from build123d import *

# Parameters (mm, degrees)
F1_DEPTH = 3
F2_R     = 5
F0_W     = 3
F0_H     = 6.5
F3_DEPTH = 7
F4_R     = 0.95
F5_DEPTH = 25
F6_R     = 1.99999


# Not quite as in the source:
# - a fillet or chamfer is up to 0.001 mm smaller than in the source, because OpenCascade refuses the exact size
# - a feature names something its author has since deleted; it is built from what else it names


with BuildPart() as f1:
    # F0 (on Top) → F1 (new body)
    with BuildSketch(Plane.XY):
        with BuildLine():
            Line((-23.06675, 0), (-28.2842712475, 0))
            Line((-28.2842712475, 0), (0, -28.2842712475))
            Line((0, -28.2842712475), (0, -23.0667636524))
            ThreePointArc((0, -23.0667636524), (-1.5, -21.5667636524), (0, -20.0667636524))
            Line((0, -20.0667636524), (0, -14.2842712475))
            Line((0, -14.2842712475), (-4.5, -14.2842712475))
            Line((-4.5, -14.2842712475), (-7.5, -14.2842712475))
            Line((-7.5, -14.2842712475), (-7.5, -7.7842712475))
            Line((-7.5, -7.7842712475), (-7.5, 0))
            Line((-7.5, 0), (-20.06675, 0))
            ThreePointArc((-20.06675, 0), (-21.56675, -1.5), (-23.06675, 0))
        make_face()
        with BuildLine():
            Line((0, -23.0667636524), (0, -28.2842712475))
            Line((0, -28.2842712475), (28.2842712475, 0))
            Line((28.2842712475, 0), (23.06675, 0))
            ThreePointArc((23.06675, 0), (21.56675, -1.5), (20.06675, 0))
            Line((20.06675, 0), (7.5, 0))
            Line((7.5, 0), (7.5, -7.7842712475))
            Line((7.5, -7.7842712475), (7.5, -14.2842712475))
            Line((7.5, -14.2842712475), (4.5, -14.2842712475))
            Line((4.5, -14.2842712475), (0, -14.2842712475))
            Line((0, -14.2842712475), (0, -20.0667636524))
            ThreePointArc((0, -20.0667636524), (1.0606601718, -20.5061034806), (1.5, -21.5667636524))
            ThreePointArc((1.5, -21.5667636524), (1.0606601718, -22.6274238242), (0, -23.0667636524))
        make_face()
        with BuildLine():
            Line((-4.2426406871, 24.0416305603), (-28.2842712475, 0))
            Line((-28.2842712475, 0), (-23.06675, 0))
            ThreePointArc((-23.06675, 0), (-21.56675, 1.5), (-20.06675, 0))
            Line((-20.06675, 0), (-7.5, 0))
            Line((-7.5, 0), (-7.5, 4.6038874425))
            Line((-7.5, 4.6038874425), (0, 4.6038874425))
            Line((0, 4.6038874425), (0, 20.0667636524))
            ThreePointArc((0, 20.0667636524), (-1.3266484173, 20.8667608118), (-1.2382102141, 22.4134250167))
            ThreePointArc((-1.2382102141, 22.4134250167), (-2.8587925726, 23.0091120056), (-4.2426406871, 24.0416305603))
        make_face()
        with BuildLine():
            ThreePointArc((0, 34.2842712475), (-5.5432771951, 30.5803718417), (-4.2426406871, 24.0416305603))
            Line((-4.2426406871, 24.0416305603), (-2.2273863607, 26.0568848867))
            ThreePointArc((-2.2273863607, 26.0568848867), (-2.9102205274, 29.4897240594), (0, 31.4342712475))
            Line((0, 31.4342712475), (0, 34.2842712475))
        make_face()
        with BuildLine():
            Line((-2.2273863607, 26.0568848867), (-4.2426406871, 24.0416305603))
            ThreePointArc((-4.2426406871, 24.0416305603), (-2.8587925726, 23.0091120056), (-1.2382102141, 22.4134250167))
            ThreePointArc((-1.2382102141, 22.4134250167), (-0.7000028406, 22.8934120697), (0, 23.0667636524))
            Line((0, 23.0667636524), (0, 25.1342712475))
            ThreePointArc((0, 25.1342712475), (-1.205452812, 25.3740507201), (-2.2273863607, 26.0568848867))
        make_face()
        with BuildLine():
            ThreePointArc((6, 28.2842712475), (4.2426406871, 32.5269119346), (0, 34.2842712475))
            Line((0, 34.2842712475), (0, 31.4342712475))
            ThreePointArc((0, 31.4342712475), (2.2273863607, 30.5116576082), (3.15, 28.2842712475))
            ThreePointArc((3.15, 28.2842712475), (2.9102205274, 27.0788184355), (2.2273863607, 26.0568848867))
            Line((2.2273863607, 26.0568848867), (4.2426406871, 24.0416305603))
            ThreePointArc((4.2426406871, 24.0416305603), (5.5432771951, 25.9881706533), (6, 28.2842712475))
        make_face()
        with BuildLine():
            ThreePointArc((1.2382102141, 22.4134250167), (2.8587925726, 23.0091120056), (4.2426406871, 24.0416305603))
            Line((4.2426406871, 24.0416305603), (2.2273863607, 26.0568848867))
            ThreePointArc((2.2273863607, 26.0568848867), (1.2054528119, 25.3740507201), (0, 25.1342712475))
            Line((0, 25.1342712475), (0, 23.0667636524))
            ThreePointArc((0, 23.0667636524), (0.7000028406, 22.8934120697), (1.2382102141, 22.4134250167))
        make_face()
        with BuildLine():
            Line((23.06675, 0), (28.2842712475, 0))
            Line((28.2842712475, 0), (4.2426406871, 24.0416305603))
            ThreePointArc((4.2426406871, 24.0416305603), (2.8587925726, 23.0091120056), (1.2382102141, 22.4134250167))
            ThreePointArc((1.2382102141, 22.4134250167), (1.4330588476, 22.0098689891), (1.5, 21.5667636524))
            ThreePointArc((1.5, 21.5667636524), (1.0606601718, 20.5061034806), (0, 20.0667636524))
            Line((0, 20.0667636524), (0, 4.6038874425))
            Line((0, 4.6038874425), (7.5, 4.6038874425))
            Line((7.5, 4.6038874425), (7.5, 0))
            Line((7.5, 0), (20.06675, 0))
            ThreePointArc((20.06675, 0), (21.56675, 1.5), (23.06675, 0))
        make_face()
    extrude(amount=F1_DEPTH)

    # F2
    f2_edges = [f1.edges().sort_by_distance(p)[0] for p in [
        (-28.284271, 0, 1.5),
        (28.284271, 0, 1.5),
        (0, -28.284271, 1.5),
        (4.242641, 24.041631, 1.5),
        (-4.242641, 24.041631, 1.5),
    ]]
    fillet(f2_edges, radius=F2_R)

    # F0 (on Top) → F3 (join)
    with BuildSketch(Plane.XY):
        with Locations((-6, -11.0342712475)):
            Rectangle(F0_W, F0_H)
        with Locations((6, -11.0342712475)):
            Rectangle(F0_W, F0_H)
    extrude(amount=F3_DEPTH)

    # F4 (on face) → F5 (cut)
    with BuildSketch(Plane(origin=(-7.5, 0, 0), x_dir=(0, -1, 0), z_dir=(-1, 0, 0))):
        with Locations((11.0342712475, 5.05)):
            Circle(F4_R)
    extrude(amount=-F5_DEPTH, mode=Mode.SUBTRACT)

    # F6 (radius 2 in the source; OpenCascade refuses exactly that, so slightly less here)
    f6_edges = [f1.edges().sort_by_distance(p)[0] for p in [
        (-6, -14.284271, 7),
        (-6, -14.284271, 3),
        (-6, -7.784271, 7),
        (-6, -7.784271, 0),
        (6, -7.784271, 0),
        (6, -14.284271, 3),
        (6, -14.284271, 7),
        (6, -7.784271, 7),
    ]]
    fillet(f6_edges, radius=F6_R)


solid = f1.part
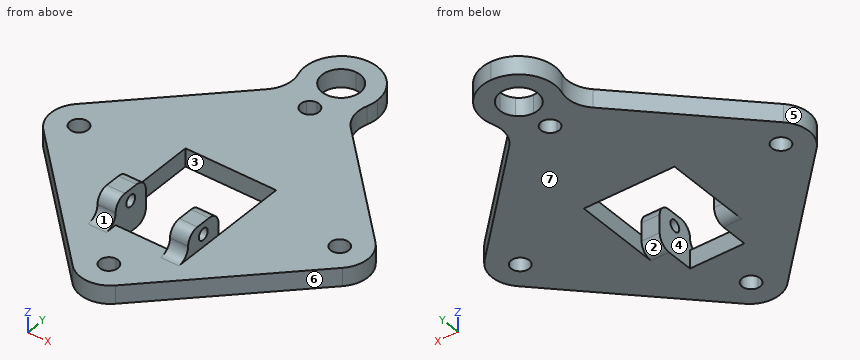
Here's how the part is built. I have some questions about the finished solid (model axes, mm). Face numbers are marked on the shaded views. A direction names the side the tool comes from. Round coordinates to 2 decimals unless told otherwise and drop trailing zeros. Loops run counter-clockwise (first coordinate to the right, second up) from the corner with the lowest first, then second, coordinate; pieces in that order, holes last.
1. If we section it at C-C on z = 0.75: Write out the boundary of the cut face in (x, y).
Answer list:
outline: (-24.75, -3.54) - (-3.54, -24.75) arc R5 ccw to (3.54, -24.75) - (24.75, -3.54) arc R5 ccw to (24.75, 3.54) - (6.93, 21.36) arc R5 cw to (5.71, 26.43) arc R6 ccw (long way) to (-5.71, 26.43) arc R5 cw to (-6.93, 21.36) - (-24.75, 3.54) arc R5 ccw to start; hole circle Ø3 at (-21.57, 0); hole (-7.5, -8.22) - (-4.5, -8.22) - (-4.5, -14.28) - (4.5, -14.28) - (4.5, -8.22) - (7.5, -8.22) - (7.5, 4.6) - (-7.5, 4.6) - close; hole circle Ø6.3 at (0, 28.28); hole circle Ø3 at (0, -21.57); hole circle Ø3 at (0, 21.57); hole circle Ø3 at (21.57, 0)
2. For P1, Ø3, axis at y = -18, z = 2, coming from the -X side; P2, Ø0.9, axis at y = -3.5, z = 1.5, coming from the +X side; P3, Ø0.9, axis at y = -1.5, z = 1.5, coming from the -X side, each with a flat end and sliding along its axis, tell me the tip position at first contact or that it passes through.
Answer list:
P1: stops at x = -11.78
P2: stops at x = 25.18
P3: stops at x = -26.1
3. If we section it at B-B on x = -13: Write out the boundary of the cut face in (y, z).
Answer list:
outline: (-15.28, 0) - (15.28, 0) - (15.28, 3) - (-15.28, 3) - close
4. If we section it at A-A on y = 0: Write out the boundary of the cut face in (x, z), plus the area to 3 significant figures.
Answer list:
outline: (-26.21, 0) - (-23.07, 0) - (-23.07, 3) - (-26.21, 3) - close; (-20.07, 0) - (-7.5, 0) - (-7.5, 3) - (-20.07, 3) - close; (7.5, 0) - (20.07, 0) - (20.07, 3) - (7.5, 3) - close; (23.07, 0) - (26.21, 0) - (26.21, 3) - (23.07, 3) - close
area: 94.3 mm2
5. If we section it at D-D on y = 16: Write out the boundary of the cut face in (x, z).
Answer list:
outline: (-12.28, 0) - (12.28, 0) - (12.28, 3) - (-12.28, 3) - close
6. Which directions (+Z, -Z, +X, -X, +Y, -Y) give clear straight access to the entire face, cutting with the end or side of a thin tool? Please do the marked faces 1, 2 and 3.
Answer list:
face 1: +Z, +X, -X, -Y
face 2: -Z
face 3: +Z, -Z
7. If I drill on line 1 along X through (y, z) = (-10, 6); line 2 along Y through (x, z) = (-1, 2.5); line 3 along Z through (x, y) = (10.5, -16), over which ranges is the centre line in solid material (lowest first)?
Answer list:
line 1: x = -7.5 to -4.5, 4.5 to 7.5
line 2: y = -26.11 to -22.68, -20.45 to -14.28, 4.6 to 20.45, 22.68 to 25.3, 31.27 to 34.2
line 3: z = 0 to 3
8. We'd pull the mould along Y, two halves only. Please class the marked faces 4, 5, 6 and 7: +Y half, -Y half, draft (parallel to the pull), parting line (faces both ways), or undercut.
Answer list:
face 4: undercut
face 5: parting line
face 6: -Y half
face 7: draft
